The listing builds one solid part. Answer for the finished solid, in the listing's coordinates (mm). Coordinates: 2 decimals unless noted, no trailing zeros. Write each loop counter-clockwise with the first axis right and the second up, starting at its lowest first coordinate (ties: lowest second). Pieces come first, ordered by that corner, then holes.
from build123d import *

# Parameters (mm, degrees)
SKETCH_W      = 50
SKETCH_H      = 10
SKETCH_R      = 1.65
SKETCH_R_2    = 1.623146
SKETCH_R_3    = 1.660457
SKETCH_R_4    = 1.568869
EXTRUDE_DEPTH = 10


with BuildPart() as part:
    # Sketch → Extrude (new body)
    with BuildSketch(Plane.XY):
        Rectangle(SKETCH_W, SKETCH_H)
        Circle(SKETCH_R, mode=Mode.SUBTRACT)
        with Locations((-10, -0.018389)):
            Circle(SKETCH_R_2, mode=Mode.SUBTRACT)
        with Locations((-19.296049, -0.018389)):
            Circle(SKETCH_R, mode=Mode.SUBTRACT)
        with Locations((10.012862, 0)):
            Circle(SKETCH_R_3, mode=Mode.SUBTRACT)
        with Locations((19.933031, 0)):
            Circle(SKETCH_R_4, mode=Mode.SUBTRACT)
    extrude(amount=EXTRUDE_DEPTH)


solid = part.part
Q1. Given pin 1 (4 mm diameter, centred on x = -10, y = -0.02, fed in from +Z), flat-ended and moving along its own axis, determine where the tip first touches the part or whether it passes through.
Answers below:
pin 1: stops at z = 10
Q2. Determine the mould class of faces 1 (the face through (0, 5, 5)), 2 (the face through (0, -5, 5)), 3 (the face through (18.366, 0.069, 4.93)) for opening direction Y: released by +Y, released by -Y, zero draft, split by the parting line, or undercut.
Answers below:
face 1: released by +Y
face 2: released by -Y
face 3: undercut
Q3. Find the intervals of material crossed by probe 1 along X at (y, z) = (-1.25, 8); probe 2 along Y at (x, z) = (20, 0.75); probe 3 along X at (y, z) = (-0.75, 1.5), in increasing order.
Answers below:
probe 1: x = -25 to -20.39, -18.2 to -11.06, -8.94 to -1.08, 1.08 to 8.92, 11.11 to 18.98, 20.88 to 25
probe 2: y = -5 to -1.57, 1.57 to 5
probe 3: x = -25 to -20.77, -17.82 to -11.45, -8.55 to -1.47, 1.47 to 8.53, 11.49 to 18.56, 21.31 to 25
Q4. The part is cut by section C-C, the plane x = 0. Write down the section's boundary in (y, z).
Answers below:
outline: (-5, 0) - (-1.65, 0) - (-1.65, 10) - (-5, 10) - close; (1.65, 0) - (5, 0) - (5, 10) - (1.65, 10) - close
Q5. The part is cut by section B-B, the plane z = 5.75. Write down the section's boundary in (x, y), then the cut area to 3 significant figures.
Answers below:
outline: (-25, -5) - (25, -5) - (25, 5) - (-25, 5) - close; hole circle Ø3.3 at (-19.3, -0.02); hole circle Ø3.25 at (-10, -0.02); hole circle Ø3.3 at (0, 0); hole circle Ø3.32 at (10.01, 0); hole circle Ø3.14 at (19.93, 0)
area: 458 mm2
Q6. The part is cut by section A-A, the plane x = -10. Write down the section's boundary in (y, z), then the cut area to 3 significant figures.
Answers below:
outline: (-5, 0) - (-1.64, 0) - (-1.64, 10) - (-5, 10) - close; (1.6, 0) - (5, 0) - (5, 10) - (1.6, 10) - close
area: 67.5 mm2
